Model file for the job. Use its own axes, mm. Coordinates: 2 decimals unless noted, no trailing zeros. Order: outer loops, then holes, each group sorted by start corner. A loop starts at its lowest first (then second) coordinate and runs counter-clockwise, first axis right, second up.
from build123d import *

# Parameters (mm, degrees)
SKETCH_1_R      = 2
SKETCH_1_R_2    = 1.5
SKETCH_1_R_3    = 65
EXTRUDE_5_DEPTH = 3


with BuildPart() as part:
    # 草图1 → 凸台-拉伸5 (new body)
    with BuildSketch(Plane.XY):
        with BuildLine():
            Line((147, 50), (178.115131306, 50))
            ThreePointArc((178.115131306, 50), (0, 185), (-178.115131306, 50))
            Line((-178.115131306, 50), (-147, 50))
            Line((-147, 50), (-147, -50))
            Line((-147, -50), (-178.115131306, -50))
            ThreePointArc((-178.115131306, -50), (0, -185), (178.115131306, -50))
            Line((178.115131306, -50), (147, -50))
            Line((147, -50), (147, 50))
        make_face()
        with Locations((-136, 8)):
            Circle(SKETCH_1_R, mode=Mode.SUBTRACT)
        with Locations((-122, 8)):
            Circle(SKETCH_1_R, mode=Mode.SUBTRACT)
        with Locations((-122, -8)):
            Circle(SKETCH_1_R, mode=Mode.SUBTRACT)
        with Locations((-136, -8)):
            Circle(SKETCH_1_R, mode=Mode.SUBTRACT)
        with Locations((122, 8)):
            Circle(SKETCH_1_R, mode=Mode.SUBTRACT)
        with Locations((136, 8)):
            Circle(SKETCH_1_R, mode=Mode.SUBTRACT)
        with Locations((136, -8)):
            Circle(SKETCH_1_R, mode=Mode.SUBTRACT)
        with Locations((122, -8)):
            Circle(SKETCH_1_R, mode=Mode.SUBTRACT)
        with Locations((14, 166)):
            Circle(SKETCH_1_R, mode=Mode.SUBTRACT)
        with Locations((14, 130)):
            Circle(SKETCH_1_R, mode=Mode.SUBTRACT)
        with Locations((-14, 130)):
            Circle(SKETCH_1_R, mode=Mode.SUBTRACT)
        with Locations((-14, 166)):
            Circle(SKETCH_1_R, mode=Mode.SUBTRACT)
        with Locations((-14, -166)):
            Circle(SKETCH_1_R, mode=Mode.SUBTRACT)
        with Locations((-14, -130)):
            Circle(SKETCH_1_R, mode=Mode.SUBTRACT)
        with Locations((14, -130)):
            Circle(SKETCH_1_R, mode=Mode.SUBTRACT)
        with Locations((14, -166)):
            Circle(SKETCH_1_R, mode=Mode.SUBTRACT)
        with Locations((-40, 165)):
            Circle(SKETCH_1_R_2, mode=Mode.SUBTRACT)
        with Locations((40, 165)):
            Circle(SKETCH_1_R_2, mode=Mode.SUBTRACT)
        with Locations((40, -120)):
            Circle(SKETCH_1_R_2, mode=Mode.SUBTRACT)
        with Locations((-40, -120)):
            Circle(SKETCH_1_R_2, mode=Mode.SUBTRACT)
        with Locations((-40, 120)):
            Circle(SKETCH_1_R_2, mode=Mode.SUBTRACT)
        with Locations((40, 120)):
            Circle(SKETCH_1_R_2, mode=Mode.SUBTRACT)
        with Locations((-40, -165)):
            Circle(SKETCH_1_R_2, mode=Mode.SUBTRACT)
        with Locations((40, -165)):
            Circle(SKETCH_1_R_2, mode=Mode.SUBTRACT)
        with Locations((-120, 60)):
            Circle(SKETCH_1_R_2, mode=Mode.SUBTRACT)
        with Locations((-120, -60)):
            Circle(SKETCH_1_R_2, mode=Mode.SUBTRACT)
        with Locations((120, -60)):
            Circle(SKETCH_1_R_2, mode=Mode.SUBTRACT)
        with Locations((120, 60)):
            Circle(SKETCH_1_R_2, mode=Mode.SUBTRACT)
        Circle(SKETCH_1_R_3, mode=Mode.SUBTRACT)
        with Locations((-75, 0)):
            Circle(SKETCH_1_R_2, mode=Mode.SUBTRACT)
        with Locations((75, 0)):
            Circle(SKETCH_1_R_2, mode=Mode.SUBTRACT)
        with Locations((-10, 75)):
            Circle(SKETCH_1_R_2, mode=Mode.SUBTRACT)
        with Locations((10, 75)):
            Circle(SKETCH_1_R_2, mode=Mode.SUBTRACT)
        with BuildLine():
            Line((-75, -102.5), (75, -102.5))
            ThreePointArc((75, -102.5), (80, -97.5), (75, -92.5))
            Line((75, -92.5), (-75, -92.5))
            ThreePointArc((-75, -92.5), (-80, -97.5), (-75, -102.5))
        make_face(mode=Mode.SUBTRACT)
        with BuildLine():
            Line((-102.5, -75), (-102.5, 75))
            ThreePointArc((-102.5, 75), (-97.5, 80), (-92.5, 75))
            Line((-92.5, 75), (-92.5, -75))
            ThreePointArc((-92.5, -75), (-97.5, -80), (-102.5, -75))
        make_face(mode=Mode.SUBTRACT)
        with BuildLine():
            Line((102.5, -75), (102.5, 75))
            ThreePointArc((102.5, 75), (97.5, 80), (92.5, 75))
            Line((92.5, 75), (92.5, -75))
            ThreePointArc((92.5, -75), (97.5, -80), (102.5, -75))
        make_face(mode=Mode.SUBTRACT)
        with BuildLine():
            Line((-75, 102.5), (75, 102.5))
            ThreePointArc((75, 102.5), (80, 97.5), (75, 92.5))
            Line((75, 92.5), (-75, 92.5))
            ThreePointArc((-75, 92.5), (-80, 97.5), (-75, 102.5))
        make_face(mode=Mode.SUBTRACT)
    extrude(amount=EXTRUDE_5_DEPTH)


solid = part.part
Q1. Cut at D-D, the plane y = 154. List the corners of the cut face in (x, z), plus the area to 3 significant figures.
Established:
outline: (-102.51, 0) - (102.51, 0) - (102.51, 3) - (-102.51, 3) - close
area: 615 mm2
Q2. Cut at A-A, the plane x = 0. List the corners of the cut face in (y, z), plus the area to 3 significant figures.
Established:
outline: (-185, 0) - (-102.5, 0) - (-102.5, 3) - (-185, 3) - close; (-92.5, 0) - (-65, 0) - (-65, 3) - (-92.5, 3) - close; (65, 0) - (92.5, 0) - (92.5, 3) - (65, 3) - close; (102.5, 0) - (185, 0) - (185, 3) - (102.5, 3) - close
area: 660 mm2
Q3. Mould opens along Y. For faces 1 (the face through (62, 19.52, 1.48)), 2 (the face through (77, 3, 3)), 3 (the face through (-3.36, -184.97, 1.48)), 4 (the face through (3.36, 184.97, 1.48)) say: pulls with the +Y half, pulls with the -Y half, needs draft (parallel to the pull), parting line crosses it, or undercut.
Established:
face 1: undercut
face 2: needs draft
face 3: pulls with the -Y half
face 4: pulls with the +Y half
Q4. Cut at C-C, the plane z = 1.7. Count the separate pieces of the cut face and the enclosed holes in it, plus the area to 3 significant figures.
Established:
separate pieces: 1
enclosed holes: 37
area: 80,500 mm2
Q5. Drop flat-ended pins along their axis: P1, Ø3.5, axis at x = 14, y = -166, coming from the -Z side; P2, Ø1.5, axis at x = -170, z = 1, coming from the -Y side; P3, Ø1, axis at x = -134.5, z = 1.5, coming from the +Y side; P4, Ø1, axis at y = 122, z = 1, coming from the +X side. Give the stop position or say it passes through.
Established:
P1: passes through
P2: stops at y = -74.7
P3: stops at y = 127.55
P4: stops at x = 139.51
Q6. Cut at B-B, the plane y = 43. List the corners of the cut face in (x, z), plus the area to 3 significant figures.
Established:
outline: (-147, 0) - (-102.5, 0) - (-102.5, 3) - (-147, 3) - close; (-92.5, 0) - (-48.74, 0) - (-48.74, 3) - (-92.5, 3) - close; (48.74, 0) - (92.5, 0) - (92.5, 3) - (48.74, 3) - close; (102.5, 0) - (147, 0) - (147, 3) - (102.5, 3) - close
area: 530 mm2
Q7. Probe line 1 (X direction, y = -120, z = 0.6); line 2 (Y direction, x = 10, z = 0.75); line 3 (Y direction, x = 48, z = 1.65). List the from-to ranges inside material, lowest first.
Established:
line 1: x = -140.8 to -41.5, -38.5 to 38.5, 41.5 to 140.8
line 2: y = -184.73 to -102.5, -92.5 to -64.23, 64.23 to 73.5, 76.5 to 92.5, 102.5 to 184.73
line 3: y = -178.66 to -102.5, -92.5 to -43.83, 43.83 to 92.5, 102.5 to 178.66
